Design review of the part built by this model. Coordinates are the model's own, in mm. A direction names the side the tool comes from. Coordinates: 2 decimals unless noted, no trailing zeros. Loops run counter-clockwise (first coordinate to the right, second up) from the corner with the lowest first, then second, coordinate; pieces in that order, holes last. Notation, with made-up numbers: (-30, 17) -> (29, 17) arc R18 cw to (29, 36) -> close; hole circle Ø8 at (-13, 23.25). An arc over 180 degrees is marked (long way). Use one line per item in the form item = value. Start each with the question number.
1. Consider section C-C (z = 1.75). State the section outline as (x, y) points.
2. Consider section A-A (x = 0). State the section outline as (y, z) points, then the cut area to 3 significant figures.
3. Machinability: for faces 5 (the face through (-4.519, 25.814, 6.526)), 6 (the face through (21.06, 2.37, -6.51)), 7 (the face through (-21.1, 3.8, -0.6)), 8 (the face through (0, 24.8, 5)), 9 (the face through (2, 25, 10)), which of the approach directions +Z, -Z, +X, -X, +Y, -Y give a long, thin tool a straight path to every point of the face, cutting with its end or side? Answer none if there is none.
4. For pin 1 (2.5 mm diameter, centred on y = 17, z = 0, fed in from -X); pin 2 (2 mm diameter, centred on x = -17, y = 23.5, fed in from +Z); pin 3 (1.8 mm diameter, centred on y = 10, z = 7, fed in from -X); pin 4 (1.5 mm diameter, centred on x = -6.5, z = 0, fed in from -Y), all flat-tipped, find the tip position at first contact; note any pin that passes through.
5. Consider section D-D (z = 5). State the section outline as (x, y) points.
6. The part is to be moulded in two halves that separate along Z. For faces 1 (the face through (21.06, 2.37, 8.49)), 2 (the face through (-20.05, 15, 0)), 3 (the face through (21.036, 0.301, 9.715)), 4 (the face through (2, 25, -10)), say which applies: released by +Z, released by -Z, zero draft, split by the parting line, or undercut.
7. Wall thickness on line 1 (Z direction, x = -21.35, y = 10); line 2 (X direction, y = 26.3, z = 0); line 3 (Z direction, x = 20.55, y = 2.5): over which ranges is each line inside the solid? List them lowest first. Write a range as from..to.
8. Consider section B-B (y = 4.5). State the section outline as (x, z) points, then the cut area to 3 significant figures.
from build123d import *

# Parameters (mm, degrees)
BOSS_EXTRU_1_DEPTH                  = 10
ESQUISSE6_R                         = 3.05
ESQUISSE6_R_2                       = 1.6
ENL_V_MAT_EXTRU_4_DEPTH             = 37.117066603
ENL_V_MAT_EXTRU_1_REACH             = 54.565
ENL_V_MAT_EXTRU_1_DIRECTION_2_DEPTH = 53.56472201
ESQUISSE4_R                         = 4.05
ENL_V_MAT_EXTRU_2_DEPTH             = 53.56472201
ENL_V_MAT_EXTRU_3_REACH             = 54.565
ESQUISSE5_R                         = 1
ENL_V_MAT_EXTRU_5_REACH             = 54.565
ESQUISSE7_R                         = 1
CONG_1_R                            = 1


with BuildPart() as part:
    # Esquisse1 → Boss.-Extru.1 (new, symmetric)
    with BuildSketch(Plane.XY):
        Polygon((-22.05, 26.8), (22.05, 26.8), (22.05, 0), (20.05, 0), (20.05, 24.8), (-20.05, 24.8), (-20.05, 0), (-22.05, 0), align=None)
    extrude(amount=BOSS_EXTRU_1_DEPTH, both=True)

    # Esquisse6 → Enlèv. mat.-Extru.4 (cut, through all)
    with BuildSketch(Plane(origin=(0, 26.8, 0), x_dir=(1, 0, 0), z_dir=(0, 1, 0))):
        with Locations(Location((0, 0, 0), (0, 0, 270))):
            Circle(ESQUISSE6_R)
        with Locations(Location((-5, 5, 0), (0, 0, 270))):
            Circle(ESQUISSE6_R_2)
        with Locations(Location((5, 5, 0), (0, 0, 270))):
            Circle(ESQUISSE6_R_2)
        with Locations(Location((5, -5, 0), (0, 0, 270))):
            Circle(ESQUISSE6_R_2)
        with Locations(Location((-5, -5, 0), (0, 0, 270))):
            Circle(ESQUISSE6_R_2)
    extrude(amount=-ENL_V_MAT_EXTRU_4_DEPTH, mode=Mode.SUBTRACT)

    # Esquisse3 → Enlèv. mat.-Extru.1 (cut, up to next)
    with BuildSketch(Plane.ZY.offset(22.05), mode=Mode.PRIVATE) as enl_v_mat_extru_1_sk1:
        with BuildLine():
            ThreePointArc((0, 0), (-7.071067812, 2.928932188), (-10, 10))
            Line((-10, 10), (-10, 0))
            Line((-10, 0), (0, 0))
        make_face()
    enl_v_mat_extru_1_tool1 = extrude(enl_v_mat_extru_1_sk1.sketch, amount=-ENL_V_MAT_EXTRU_1_REACH, mode=Mode.PRIVATE) & part.part
    # Esquisse3 → Enlèv. mat.-Extru.1 (cut, up to next)
    with BuildSketch(Plane.ZY.offset(22.05), mode=Mode.PRIVATE) as enl_v_mat_extru_1_sk2:
        with BuildLine():
            ThreePointArc((10, 10), (7.071067812, 2.928932188), (0, 0))
            Line((0, 0), (10, 0))
            Line((10, 0), (10, 10))
        make_face()
    enl_v_mat_extru_1_tool2 = extrude(enl_v_mat_extru_1_sk2.sketch, amount=-ENL_V_MAT_EXTRU_1_REACH, mode=Mode.PRIVATE) & part.part
    add(enl_v_mat_extru_1_tool1.solids().sort_by_distance((-22.05, 2.233679, -7.766321))[0], mode=Mode.SUBTRACT)
    add(enl_v_mat_extru_1_tool2.solids().sort_by_distance((-22.05, 2.233679, 7.766321))[0], mode=Mode.SUBTRACT)

    # Esquisse3 → Enlèv. mat.-Extru.1 direction 2 (cut)
    with BuildSketch(Plane.ZY.offset(22.05)):
        with BuildLine():
            ThreePointArc((0, 0), (-7.071067812, 2.928932188), (-10, 10))
            Line((-10, 10), (-10, 0))
            Line((-10, 0), (0, 0))
        make_face()
        with BuildLine():
            ThreePointArc((10, 10), (7.071067812, 2.928932188), (0, 0))
            Line((0, 0), (10, 0))
            Line((10, 0), (10, 10))
        make_face()
    extrude(amount=ENL_V_MAT_EXTRU_1_DIRECTION_2_DEPTH, mode=Mode.SUBTRACT)

    # Esquisse4 → Enlèv. mat.-Extru.2 (cut, through all)
    with BuildSketch(Plane.ZY.offset(22.05)):
        with Locations(Location((0, 10, 0), (0, 0, 270))):
            Circle(ESQUISSE4_R)
    extrude(amount=-ENL_V_MAT_EXTRU_2_DEPTH, mode=Mode.SUBTRACT)

    # Esquisse5 → Enlèv. mat.-Extru.3 (cut, up to next)
    with BuildSketch(Plane.ZY.offset(22.05), mode=Mode.PRIVATE) as enl_v_mat_extru_3_sk1:
        with Locations(Location((-7, 10, 0), (0, 0, 270))):
            Circle(ESQUISSE5_R)
    enl_v_mat_extru_3_tool1 = extrude(enl_v_mat_extru_3_sk1.sketch, amount=-ENL_V_MAT_EXTRU_3_REACH, mode=Mode.PRIVATE) & part.part
    # Esquisse5 → Enlèv. mat.-Extru.3 (cut, up to next)
    with BuildSketch(Plane.ZY.offset(22.05), mode=Mode.PRIVATE) as enl_v_mat_extru_3_sk2:
        with Locations(Location((0, 17, 0), (0, 0, 270))):
            Circle(ESQUISSE5_R)
    enl_v_mat_extru_3_tool2 = extrude(enl_v_mat_extru_3_sk2.sketch, amount=-ENL_V_MAT_EXTRU_3_REACH, mode=Mode.PRIVATE) & part.part
    # Esquisse5 → Enlèv. mat.-Extru.3 (cut, up to next)
    with BuildSketch(Plane.ZY.offset(22.05), mode=Mode.PRIVATE) as enl_v_mat_extru_3_sk3:
        with Locations(Location((7, 10, 0), (0, 0, 270))):
            Circle(ESQUISSE5_R)
    enl_v_mat_extru_3_tool3 = extrude(enl_v_mat_extru_3_sk3.sketch, amount=-ENL_V_MAT_EXTRU_3_REACH, mode=Mode.PRIVATE) & part.part
    # Esquisse5 → Enlèv. mat.-Extru.3 (cut, up to next)
    with BuildSketch(Plane.ZY.offset(22.05), mode=Mode.PRIVATE) as enl_v_mat_extru_3_sk4:
        with Locations(Location((0, 3, 0), (0, 0, 270))):
            Circle(ESQUISSE5_R)
    enl_v_mat_extru_3_tool4 = extrude(enl_v_mat_extru_3_sk4.sketch, amount=-ENL_V_MAT_EXTRU_3_REACH, mode=Mode.PRIVATE) & part.part
    add(enl_v_mat_extru_3_tool1.solids().sort_by_distance((-22.05, 10, -7))[0], mode=Mode.SUBTRACT)
    add(enl_v_mat_extru_3_tool2.solids().sort_by_distance((-22.05, 17, 0))[0], mode=Mode.SUBTRACT)
    add(enl_v_mat_extru_3_tool3.solids().sort_by_distance((-22.05, 10, 7))[0], mode=Mode.SUBTRACT)
    add(enl_v_mat_extru_3_tool4.solids().sort_by_distance((-22.05, 3, 0))[0], mode=Mode.SUBTRACT)

    # Esquisse7 → Enlèv. mat.-Extru.5 (cut, up to next)
    with BuildSketch(Plane(origin=(22.05, 0, 0), x_dir=(0, 0, -1), z_dir=(1, 0, 0)), mode=Mode.PRIVATE) as enl_v_mat_extru_5_sk1:
        with Locations(Location((-7.5, 2.5, 0), (0, 0, 90))):
            Circle(ESQUISSE7_R)
    enl_v_mat_extru_5_tool1 = extrude(enl_v_mat_extru_5_sk1.sketch, amount=-ENL_V_MAT_EXTRU_5_REACH, mode=Mode.PRIVATE) & part.part
    # Esquisse7 → Enlèv. mat.-Extru.5 (cut, up to next)
    with BuildSketch(Plane(origin=(22.05, 0, 0), x_dir=(0, 0, -1), z_dir=(1, 0, 0)), mode=Mode.PRIVATE) as enl_v_mat_extru_5_sk2:
        with Locations(Location((7.5, 2.5, 0), (0, 0, 90))):
            Circle(ESQUISSE7_R)
    enl_v_mat_extru_5_tool2 = extrude(enl_v_mat_extru_5_sk2.sketch, amount=-ENL_V_MAT_EXTRU_5_REACH, mode=Mode.PRIVATE) & part.part
    # Esquisse7 → Enlèv. mat.-Extru.5 (cut, up to next)
    with BuildSketch(Plane(origin=(22.05, 0, 0), x_dir=(0, 0, -1), z_dir=(1, 0, 0)), mode=Mode.PRIVATE) as enl_v_mat_extru_5_sk3:
        with Locations(Location((7.5, 17.5, 0), (0, 0, 90))):
            Circle(ESQUISSE7_R)
    enl_v_mat_extru_5_tool3 = extrude(enl_v_mat_extru_5_sk3.sketch, amount=-ENL_V_MAT_EXTRU_5_REACH, mode=Mode.PRIVATE) & part.part
    # Esquisse7 → Enlèv. mat.-Extru.5 (cut, up to next)
    with BuildSketch(Plane(origin=(22.05, 0, 0), x_dir=(0, 0, -1), z_dir=(1, 0, 0)), mode=Mode.PRIVATE) as enl_v_mat_extru_5_sk4:
        with Locations(Location((-7.5, 17.5, 0), (0, 0, 90))):
            Circle(ESQUISSE7_R)
    enl_v_mat_extru_5_tool4 = extrude(enl_v_mat_extru_5_sk4.sketch, amount=-ENL_V_MAT_EXTRU_5_REACH, mode=Mode.PRIVATE) & part.part
    add(enl_v_mat_extru_5_tool1.solids().sort_by_distance((22.05, 2.5, 7.5))[0], mode=Mode.SUBTRACT)
    add(enl_v_mat_extru_5_tool2.solids().sort_by_distance((22.05, 2.5, -7.5))[0], mode=Mode.SUBTRACT)
    add(enl_v_mat_extru_5_tool3.solids().sort_by_distance((22.05, 17.5, -7.5))[0], mode=Mode.SUBTRACT)
    add(enl_v_mat_extru_5_tool4.solids().sort_by_distance((22.05, 17.5, 7.5))[0], mode=Mode.SUBTRACT)

    # Congé1
    cong_1_edges = [part.edges().sort_by_distance(p)[0] for p in [
        (21.05, 0, 10),
        (21.05, 0, -10),
    ]]
    fillet(cong_1_edges, radius=CONG_1_R)


solid = part.part
Geometry check:
q1.outline = (-22.05, 0.15) -> (-20.05, 0.15) -> (-20.05, 6.35) -> (-22.05, 6.35) -> close; (-22.05, 13.65) -> (-20.05, 13.65) -> (-20.05, 24.8) -> (-2.5, 24.8) -> (-2.5, 26.8) -> (-22.05, 26.8) -> close; (2.5, 24.8) -> (20.05, 24.8) -> (20.05, 13.65) -> (22.05, 13.65) -> (22.05, 26.8) -> (2.5, 26.8) -> close; (20.05, 0) -> (22.05, 0) -> (22.05, 6.35) -> (20.05, 6.35) -> close
q2.outline = (24.8, -10) -> (26.8, -10) -> (26.8, -3.05) -> (24.8, -3.05) -> close; (24.8, 3.05) -> (26.8, 3.05) -> (26.8, 10) -> (24.8, 10) -> close
q2.area = 27.8 mm²
q3.face_5 = +Y, -Y
q3.face_6 = +X
q3.face_7 = -X
q3.face_8 = +Z, -Z, -Y
q3.face_9 = +Z, +X, -X, +Y, -Y
q4.pin_1 = -22.05
q4.pin_2 = through
q4.pin_3 = 20.05
q4.pin_4 = 24.8
q5.outline = (-22.05, 1.34) -> (-20.05, 1.34) -> (-20.05, 24.8) -> (-6.6, 24.8) -> (-6.6, 26.8) -> (-22.05, 26.8) -> close; (-3.4, 24.8) -> (3.4, 24.8) -> (3.4, 26.8) -> (-3.4, 26.8) -> close; (6.6, 24.8) -> (20.05, 24.8) -> (20.05, 0) -> (22.05, 0) -> (22.05, 26.8) -> (6.6, 26.8) -> close
q6.face_1 = undercut
q6.face_2 = zero draft
q6.face_3 = released by +Z
q6.face_4 = released by -Z
q7.line_1 = -10..-8, -6..-4.05, 4.05..6, 8..10
q7.line_2 = -22.05..-3.05, 3.05..22.05
q7.line_3 = -10..-8.5, -6.5..6.5, 8.5..10
q8.outline = (-22.05, -8.35) -> (-20.05, -8.35) -> (-20.05, 8.35) -> (-22.05, 8.35) -> close; (20.05, -10) -> (22.05, -10) -> (22.05, 10) -> (20.05, 10) -> close
q8.area = 73.4 mm²
